Geometry check sheet. Reference: the model listing, model coordinates, mm. Coordinates: 2 decimals unless noted, no trailing zeros. Order: outer loops, then holes, each group sorted by start corner. A loop starts at its lowest first (then second) coordinate and runs counter-clockwise, first axis right, second up. Notation, with made-up numbers: (-35.75, -2) - (-30.75, -2) arc R29 ccw to (-30.75, 26) - close; hole circle Ø7 at (12, -9.75). An arc over 180 degrees is marked (long way). Put each result on its own line as item: value.
from build123d import *

# Parameters (mm, degrees)
BOSS_EXTRUDE1_DEPTH      = 300
BOSS_EXTRUDE1_DEPTH_BACK = 500
SKETCH2_R                = 75
CIRPATTERN1_COUNT        = 3


with BuildPart() as part:
    # Sketch1 → Revolve1 (revolve)
    with BuildSketch(Plane(origin=(0, 0, 0), x_dir=(1, 0, 0), z_dir=(0, 1, 0))):
        with BuildLine():
            Line((-750, 750), (-750, 677.44666419))
            ThreePointArc((-750, 677.44666419), (-943.246815965, 362.931711199), (-1010.66017178, 0))
            Line((-1010.66017178, 0), (-1060.66017178, 0))
            ThreePointArc((-1060.66017178, 0), (-979.922223657, 405.89707511), (-750, 750))
        make_face()
    revolve(axis=Axis((-1110.59399243, 0, 0), (1, 0, 0)))

    # Sketch2 → Boss-Extrude1 (add, two sides: drawn at the far end of the back side and taken through both)
    with BuildSketch(Plane(origin=(-750, 0, 0), x_dir=(0, 0, -1), z_dir=(1, 0, 0)).offset(-BOSS_EXTRUDE1_DEPTH_BACK)):
        with Locations(Location((0, 0, 0), (0, 0, 180))):
            Circle(SKETCH2_R)
    extrude(amount=BOSS_EXTRUDE1_DEPTH + BOSS_EXTRUDE1_DEPTH_BACK)

    # Sketch5 → Revolve2 (revolve)
    with BuildSketch(Plane.XY):
        Polygon((-450, 75), (-881.052293811, 506.052293811), (-899.012806053, 488.091781569), (-467.960512242, 57.039487758), align=None)
    revolve2 = revolve(axis=Axis((-467.960512242, 57.039487758, 0), (-0.7071067811865465, 0.7071067811865487, 0)))

    # CirPattern1: Revolve2 ×3 about axis
    cirpattern1_axis = Axis((-450, 0, 0), (1, 0, 0))
    for i in range(1, CIRPATTERN1_COUNT):
        add(revolve2.rotate(cirpattern1_axis, i * 360 / CIRPATTERN1_COUNT))


solid = part.part
Q1. Section check A-A on x = -935. Record the boundary of the cut face in (y, z), then the cut area to 3 significant figures.
Answer block:
outline: circle Ø1001.55 at (0, 0); circle Ø150 at (0, 0); hole circle Ø767.36 at (0, 0)
area: 343,000 mm^2
Q2. Draft check along Z on faces 1 (the flat face through (-1250, -1, -1)), 2 (the cylindrical face through (-732.842, -22.528, 71.537)), 3 (the cylindrical face through (-1155.347, 66.538, 34.608)). Enter one of: pulls with the +Z half, pulls with the -Z half, needs draft (parallel to the pull), parting line crosses it, or undercut.
Answer block:
face 1: needs draft
face 2: undercut
face 3: parting line crosses it
Q3. Section check C-C on y = -601. Record the boundary of the cut face in (x, z).
Answer block:
outline: (-750, -448.66) - (-750, -312.62) arc R812.55 cw to (-750, 312.62) - (-750, 448.66) arc R873.96 ccw to start
Q4. Section check B-B on x = -831. State how many separate pieces and enclosed holes the cut face has, then the cut area to 3 significant figures.
Answer block:
separate pieces: 5
enclosed holes: 1
area: 352,000 mm^2
Q5. Depth check by flat-ended pin: pin 1 Ø1 at (y, z) = (-96.5, -246) entering from +X; pin 2 Ø12 at (y, z) = (532, -96.5) entering from +X; pin 3 Ø4 at (x, y) = (-792, -236.5) entering from -Z. Enter the tip coordinate at first touch or a pass-through.
Answer block:
pin 1: stops at x = -975.37
pin 2: stops at x = -850.04
pin 3: stops at z = -667.16
Q6. Thickness scan on L1, parallel to X at y = -130, z = -265; L2, parallel to Z at x = -672, y = -139; L3, parallel to Y at x = -824, z = 166. Record the ranges inside material, lowest first. Write a range as [from, to].
Answer block:
L1: x = [-1018.76, -966.6], [-727.71, -683.12]
L2: z = [-259.7, -198.36], [198.36, 259.7]
L3: y = [-646.89, -561.16], [561.16, 646.89]
Q7. Section check D-D on z = 631.5. Record the boundary of the cut face in (x, y), then the cut area to 3 significant figures.
Answer block:
outline: (-750, -404.61) - (-750, -245.24) arc R789.08 cw to (-750, 245.24) - (-750, 404.61) arc R852.18 ccw to start
area: 43,000 mm^2
